For this review, use the dimensioned drawing (mm, ordinates from the lowest corner) and the shaded views. A direction names the side the tool comes from. Give positions to 0.01 mm unless a question says otherwise; leave off trailing zeros. Write each loop counter-clockwise with the first axis right and the second up, starting at its lowest first coordinate (ties: lowest second). Pieces come first, ordered by that corner, then holes. Notation, with made-up numbers: (66, 39.25) -> (95, 39.25) arc R33 ccw to (95, 78.25) -> close; hole circle Ø6 at (59.25, -37). An arc over 180 degrees is marked (long way). Write each question's results on one line, items separated by ' | '. Start each with the question number.
(1) Take a section at A-A (z = 3.25). State the section outline as (x, y) points.
(2) Clearance check with flat-ended pins moving along their axes: pin 1 (3.5 mm diameter, centred on x = 4.9, y = 5, fed in from -Z); pin 2 (1.5 mm diameter, centred on x = 33, z = 3.5, fed in from -Y); pin 3 (2 mm diameter, centred on x = 6.5, y = 16, fed in from +Z). State where each tip first meets the part, or that it passes through.
(3) Take a section at C-C (y = 25). State the section outline as (x, z) points.
(4) To check wall thickness, follow probe 1 along Y at (x, z) = (4.9, 2.5); probe 2 along Y at (x, z) = (25, 0.9); probe 3 along Y at (x, z) = (41.5, 4). State the ranges of each line that lie inside material, in increasing order.
(5) Take a section at D-D (x = 4.9). State the section outline as (y, z) points.
(6) For the marked faces 5, 6 and 7, list the 3-axis set-ups (+Z, -Z, +X, -X, +Y, -Y) from which the entire face can be reached by the end or side of a thin tool; tool diameter is ignored.
(7) Mouldability with a two-part tool opening along Y and no side actions: class the marked faces 1, 2, 3 and 4 as released by +Y, released by -Y, zero draft, split by the parting line, or undercut.
(8) Take a section at B-B (x = 16). State the section outline as (y, z) points, plus the area to 3 significant figures.
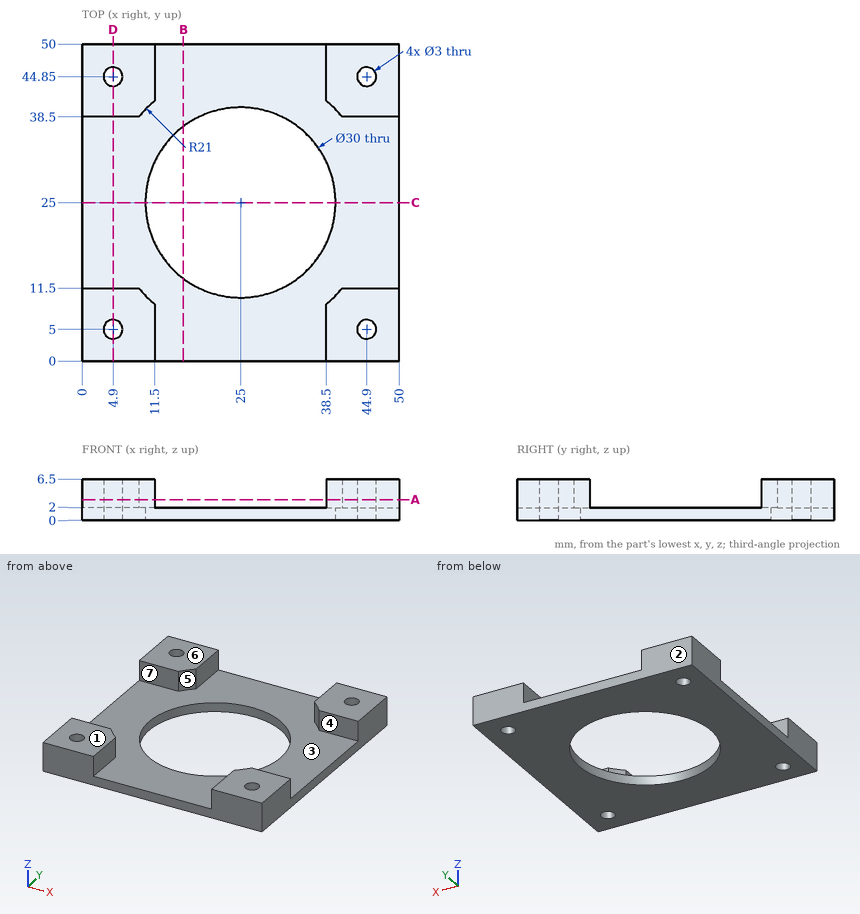
Report:
1) outline: (0, 0) -> (11.5, 0) -> (11.5, 8.91) arc R21 cw to (8.91, 11.5) -> (0, 11.5) -> close; (0, 38.5) -> (8.91, 38.5) arc R21 cw to (11.5, 41.09) -> (11.5, 50) -> (0, 50) -> close; (38.5, 0) -> (50, 0) -> (50, 11.5) -> (41.09, 11.5) arc R21 cw to (38.5, 8.91) -> close; (38.5, 41.09) arc R21 cw to (41.09, 38.5) -> (50, 38.5) -> (50, 50) -> (38.5, 50) -> close; hole circle Ø3 at (4.9, 5); hole circle Ø3 at (4.9, 44.85); hole circle Ø3 at (44.9, 5); hole circle Ø3 at (44.9, 44.85)
2) pin 1: z = 0 | pin 2: through | pin 3: z = 2
3) outline: (0, 0) -> (10, 0) -> (10, 2) -> (0, 2) -> close; (40, 0) -> (50, 0) -> (50, 2) -> (40, 2) -> close
4) probe 1: 0 to 3.5, 6.5 to 11.5, 38.5 to 43.35, 46.35 to 50 | probe 2: 0 to 10, 40 to 50 | probe 3: 0 to 11.5, 38.5 to 50
5) outline: (0, 0) -> (3.5, 0) -> (3.5, 6.5) -> (0, 6.5) -> close; (6.5, 0) -> (43.35, 0) -> (43.35, 6.5) -> (38.5, 6.5) -> (38.5, 2) -> (11.5, 2) -> (11.5, 6.5) -> (6.5, 6.5) -> close; (46.35, 0) -> (50, 0) -> (50, 6.5) -> (46.35, 6.5) -> close
6) face 5: +Z | face 6: +Z, +X, -X, +Y, -Y | face 7: +Z, +X, -X
7) face 1: zero draft | face 2: released by +Y | face 3: undercut | face 4: undercut
8) outline: (0, 0) -> (13, 0) -> (13, 2) -> (0, 2) -> close; (37, 0) -> (50, 0) -> (50, 2) -> (37, 2) -> close | area: 52.0 mm2
